Source: CAD feature listing. Evaluate the final solid. Frame: model axes, mm. A direction names the side the tool comes from. Coordinates: 2 decimals unless noted, no trailing zeros. Write each loop counter-clockwise with the first axis right and the second up, starting at its lowest first coordinate (ties: lowest second). Pieces come first, ordered by that corner, then holes. Notation, with made-up numbers: (63.25, -16.75) - (91.25, -16.75) arc R12 cw to (91.25, -10.75) - close; hole circle Ø11 at (-17.75, 30.5). An arc over 180 degrees is marked (long way). One line per item, written item: value.
from build123d import *

# Parameters (mm, degrees)
SKETCH1_R           = 4.82
BOSS_EXTRUDE1_DEPTH = 7.7
SKETCH2_R           = 5.65
BOSS_EXTRUDE2_DEPTH = 1.5
SKETCH3_R           = 4.075
BOSS_EXTRUDE3_DEPTH = 28.5
SKETCH4_R           = 3
CUT_EXTRUDE1_DEPTH  = 39.537449319
SKETCH5_R           = 3.95
CUT_EXTRUDE2_DEPTH  = 7.7
SKETCH6_W           = 4.15
SKETCH6_H           = 2.4
CUT_EXTRUDE3_DEPTH  = 7.7


with BuildPart() as part:
    # Sketch1 → Boss-Extrude1 (new body)
    with BuildSketch(Plane(origin=(0, 0, 0), x_dir=(0, 0, -1), z_dir=(1, 0, 0))):
        with Locations(Location((0, 0, 0), (0, 0, 180))):
            Circle(SKETCH1_R)
    extrude(amount=BOSS_EXTRUDE1_DEPTH)

    # Sketch2 → Boss-Extrude2 (add)
    with BuildSketch(Plane(origin=(7.7, 0, 0), x_dir=(0, 0, -1), z_dir=(1, 0, 0))):
        Circle(SKETCH2_R)
    extrude(amount=BOSS_EXTRUDE2_DEPTH)

    # Sketch3 → Boss-Extrude3 (add)
    with BuildSketch(Plane(origin=(9.2, 0, 0), x_dir=(0, 0, -1), z_dir=(1, 0, 0))):
        with Locations(Location((0, 0, 0), (0, 0, 180))):
            Circle(SKETCH3_R)
    extrude(amount=BOSS_EXTRUDE3_DEPTH)

    # Sketch4 → Cut-Extrude1 (cut, through all)
    with BuildSketch(Plane(origin=(37.7, 0, 0), x_dir=(0, 0, -1), z_dir=(1, 0, 0))):
        Circle(SKETCH4_R)
    extrude(amount=-CUT_EXTRUDE1_DEPTH, mode=Mode.SUBTRACT)

    # Sketch5 → Cut-Extrude2 (cut)
    with BuildSketch(Plane.ZY):
        Circle(SKETCH5_R)
    extrude(amount=-CUT_EXTRUDE2_DEPTH, mode=Mode.SUBTRACT)

    # Sketch6 → Cut-Extrude3 (cut)
    with BuildSketch(Plane(origin=(0, 0, 0), x_dir=(1, 0, 0), z_dir=(0, 1, 0))):
        with Locations((17.875, 0)):
            Rectangle(SKETCH6_W, SKETCH6_H)
    extrude(amount=CUT_EXTRUDE3_DEPTH, mode=Mode.SUBTRACT)


solid = part.part
1) Section query D-D on y = -1.5. Output: boundary loops of the cut face in (x, z).
Values found:
outline: (0, -4.58) - (7.7, -4.58) - (7.7, -5.45) - (9.2, -5.45) - (9.2, -3.79) - (37.7, -3.79) - (37.7, -2.6) - (7.7, -2.6) - (7.7, -3.65) - (0, -3.65) - close; (0, 3.65) - (7.7, 3.65) - (7.7, 2.6) - (37.7, 2.6) - (37.7, 3.79) - (9.2, 3.79) - (9.2, 5.45) - (7.7, 5.45) - (7.7, 4.58) - (0, 4.58) - close
2) Section query C-C on x = 5.5. Output: boundary loops of the cut face in (y, z).
Values found:
outline: circle Ø9.64 at (0, 0); hole circle Ø7.9 at (0, 0)
3) Contact query for flat-ended pins moving along their axis: P1, Ø2, axis at x = 4.5, y = -1, coming from the -Z side; P2, Ø3, axis at x = 32.5, y = 0.5, coming from the +Z side (3 decimals); P3, Ø0.7, axis at y = 3, z = 0, coming from the -X side. Output: stop coordinate, or through.
Values found:
P1: z = -4.82
P2: z = 4.075
P3: x = 7.7
4) Reachability of faces 4 (the cylindrical face through (22.91, -2.93, 0.65)), 5 (the flat face through (9.2, -4, -2)), 6 (the flat face through (7.7, 3, -1)), 7 (the flat face through (18, 3, 1.2)), 8 (the flat face through (0, -4, -1)) from +Z, -Z, +X, -X, +Y, -Y: full face, straight path, thin tool, end or side. Return the list, or none.
Values found:
face 4: +X, -X
face 5: +X
face 6: -X
face 7: +Y
face 8: +Z, -Z, -X, +Y, -Y
5) Draft query along Z for faces 1 (the flat face through (37.7, 3, -2)), 2 (the flat face through (15.8, 3.4, 0)), 3 (the cylindrical face through (23.25, -3.436, 2.191)). Return one class per face: released by +Z, released by -Z, zero draft, split by the parting line, or undercut.
Values found:
face 1: zero draft
face 2: undercut
face 3: split by the parting line
6) Section query A-A on z = 0. Output: boundary loops of the cut face in (x, y) (3 decimals), then the cut area to 3 significant figures.
Values found:
outline: (0, -4.82) - (7.7, -4.82) - (7.7, -5.65) - (9.2, -5.65) - (9.2, -4.075) - (37.7, -4.075) - (37.7, -3) - (7.7, -3) - (7.7, -3.95) - (0, -3.95) - close; (0, 3.95) - (7.7, 3.95) - (7.7, 3) - (15.8, 3) - (15.8, 4.075) - (9.2, 4.075) - (9.2, 5.65) - (7.7, 5.65) - (7.7, 4.82) - (0, 4.82) - close; (19.95, 3) - (37.7, 3) - (37.7, 4.075) - (19.95, 4.075) - close
area: 78.2 mm2
7) Section query B-B on y = 0. Output: boundary loops of the cut face in (x, z) (3 decimals), then the cut area to 3 significant figures.
Values found:
outline: (0, -4.82) - (7.7, -4.82) - (7.7, -5.65) - (9.2, -5.65) - (9.2, -4.075) - (37.7, -4.075) - (37.7, -3) - (7.7, -3) - (7.7, -3.95) - (0, -3.95) - close; (0, 3.95) - (7.7, 3.95) - (7.7, 3) - (37.7, 3) - (37.7, 4.075) - (9.2, 4.075) - (9.2, 5.65) - (7.7, 5.65) - (7.7, 4.82) - (0, 4.82) - close
area: 82.6 mm2
8) Material intervals for line 1 (X direction, y = 3.5, z = -0.5); line 2 (Y direction, x = 31, z = 0) (3 decimals); line 3 (Y direction, x = 3.25, z = 0), sorted ascending.
Values found:
line 1: 7.7 to 15.8, 19.95 to 37.7
line 2: -4.075 to -3, 3 to 4.075
line 3: -4.82 to -3.95, 3.95 to 4.82
